Answer from the drawing. Dimensions are ordinates in mm from the lowest x, y and z of the part. A direction names the side the tool comes from. Coordinates: 2 decimals unless noted, no trailing zeros. Order: outer loops, then holes, each group sorted by start corner. A loop starts at its lowest first (then second) coordinate and runs counter-clockwise, first axis right, second up.
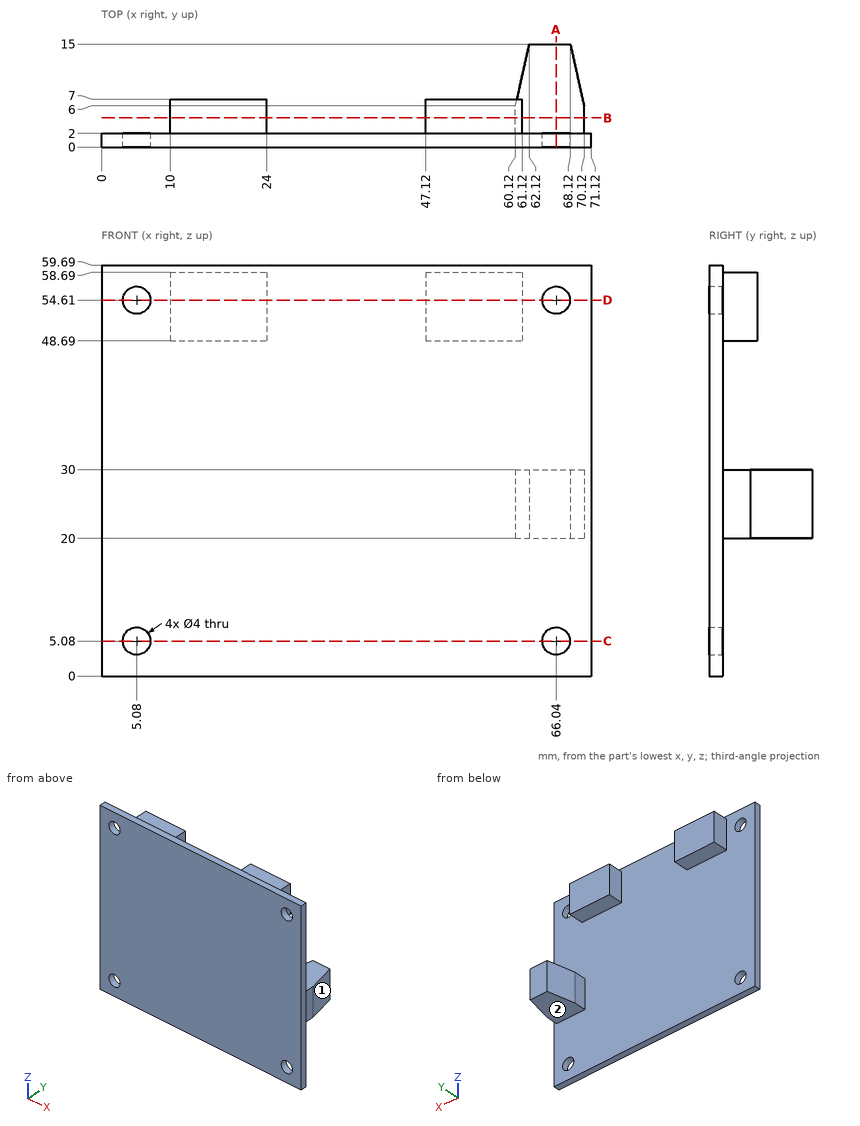
1) Section D-D (z = 54.61) is taken. Give the vertices of the cut face in (x, y), then the cut area to 3 significant figures.
2) Each of these flat-tipped pins is pushed along its axis until it touches: P1, Ø1.5, axis at x = 14, y = 5, coming from the -Z side; P2, Ø2, axis at x = 16, z = 33, coming from the +Y side; P3, Ø2.5, axis at x = 5.08, z = 54.61, coming from the -Y side; P4, Ø4, axis at x = 49.5, z = 52.5, coming from the +Y side. Where does it stop, or does it pass through?
3) Section B-B (y = 4.25) is taken. Give the vertices of the cut face in (x, z).
4) A tool of negligible diameter and unlimited length cuts with its end or side. For the marked faces 1 and 2, from which of +Z, -Z, +X, -X, +Y, -Y can it reach the whole face along a straight path? Write none if from no direction.
5) Section C-C (z = 5.08) is taken. Give the vertices of the cut face in (x, y), then the cut area to 3 significant figures.
6) Consider L1, parallel to Z at x = 5.08, y = 0.95; L2, parallel to X at y = 1.2, z = 5.08; L3, parallel to X at y = 4.5, z = 50. Determine where each line is inside the solid, lowest interval first.
7) Section A-A (x = 66.04) is taken. Give the vertices of the cut face in (y, z).
Filled sheet:
1. outline: (0, 0) - (3.08, 0) - (3.08, 2) - (0, 2) - close; (7.08, 0) - (64.04, 0) - (64.04, 2) - (61.12, 2) - (61.12, 7) - (47.12, 7) - (47.12, 2) - (24, 2) - (24, 7) - (10, 7) - (10, 2) - (7.08, 2) - close; (68.04, 0) - (71.12, 0) - (71.12, 2) - (68.04, 2) - close
1. area: 266 mm2
2. P1: stops at z = 48.69
2. P2: stops at y = 2
2. P3: passes through
2. P4: stops at y = 7
3. outline: (10, 48.69) - (24, 48.69) - (24, 58.69) - (10, 58.69) - close; (47.12, 48.69) - (61.12, 48.69) - (61.12, 58.69) - (47.12, 58.69) - close; (60.12, 20) - (70.12, 20) - (70.12, 30) - (60.12, 30) - close
4. face 1: +Z, -Z, +X, +Y
4. face 2: -Z, +X, -X, +Y
5. outline: (0, 0) - (3.08, 0) - (3.08, 2) - (0, 2) - close; (7.08, 0) - (64.04, 0) - (64.04, 2) - (7.08, 2) - close; (68.04, 0) - (71.12, 0) - (71.12, 2) - (68.04, 2) - close
5. area: 126 mm2
6. L1: z = 0 to 3.08, 7.08 to 52.61, 56.61 to 59.69
6. L2: x = 0 to 3.08, 7.08 to 64.04, 68.04 to 71.12
6. L3: x = 10 to 24, 47.12 to 61.12
7. outline: (0, 0) - (2, 0) - (2, 3.08) - (0, 3.08) - close; (0, 7.08) - (2, 7.08) - (2, 20) - (15, 20) - (15, 30) - (2, 30) - (2, 52.61) - (0, 52.61) - close; (0, 56.61) - (2, 56.61) - (2, 59.69) - (0, 59.69) - close
